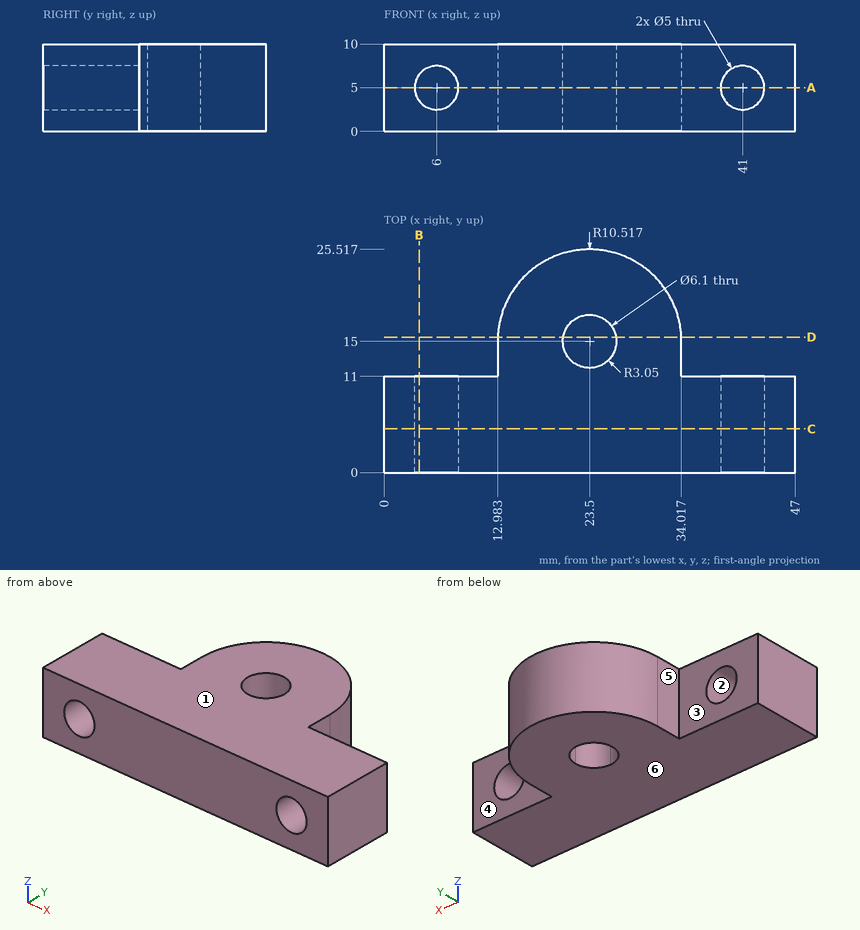
Geometry check sheet. Reference: drawing and pictorial views, mm from the part's lowest x, y, z. A direction names the side the tool comes from. Give positions to 0.01 mm unless a question says otherwise; leave off trailing zeros. Order: outer loops, then holes, each group sorted by start corner. A loop starts at its lowest first (then second) coordinate and runs counter-clockwise, first axis right, second up. Notation, with made-up numbers: (31.25, 68) -> (61.25, 68) arc R11 ccw to (61.25, 88) -> close; hole circle Ø2 at (12, -14). An arc over 180 degrees is marked (long way). Use CSV: the item, a comma, the result in double quotes. Start each with the question number.
1) Sectioned sample at D-D, the plane y = 15.5. Record the boundary of the cut face in (x, z) (1 decimal), plus the area to 3 significant figures.
2) Material ranges on line 1 (X direction, y = 8, z = 5); line 2 (X direction, y = 15, z = 7.25); line 3 (Y direction, x = 23.5, z = 8.25), recorded low to high. Write a range as from..to.
3) Sectioned sample at A-A, the plane z = 5. Give the number of separate pieces and of enclosed holes in the cut face, plus the area to 3 significant figures.
4) Sectioned sample at C-C, the plane y = 5. Record the boundary of the cut face in (x, z).
5) Mould release check, pull along Z, two halves, no side actions. Record for the marked faces 1, 2 and 3: released by +Z, released by -Z, zero draft, split by the parting line, or undercut.
6) Set-up check for the marked faces 4, 5 and 6: record each of +Z, -Z, +X, -X, +Y, -Y from which the full face is reachable in a straight line by a thin tool's end or side.
7) Go/stop test with flat-tipped pins: P1, Ø1.5, axis at y = 17, z = 4, coming from the -X side; P2, Ø5, axis at x = 43, z = 7.5, coming from the +Y side; P3, Ø2, axis at y = 12.5, z = 5.5, coming from the -X side. Record where each tip stops, or that it passes through.
8) Sectioned sample at B-B, the plane x = 4. Record the boundary of the cut face in (y, z), plus the area to 3 significant figures.
Recorded:
1,outline,"(13, 0) -> (20.5, 0) -> (20.5, 10) -> (13, 10) -> close; (26.5, 0) -> (34, 0) -> (34, 10) -> (26.5, 10) -> close"
1,area,"150 mm2"
2,line 1,"0..3.5, 8.5..38.5, 43.5..47"
2,line 2,"12.98..20.45, 26.55..34.02"
2,line 3,"0..11.95, 18.05..25.52"
3,separate pieces,"3"
3,enclosed holes,"1"
3,area,"636 mm2"
4,outline,"(0, 0) -> (47, 0) -> (47, 10) -> (0, 10) -> close; hole circle Ø5 at (6, 5); hole circle Ø5 at (41, 5)"
5,face 1,"released by +Z"
5,face 2,"undercut"
5,face 3,"zero draft"
6,face 4,"+Z, -Z, +X, +Y"
6,face 5,"+Z, -Z, -X, +Y"
6,face 6,"-Z, +X, -X, +Y, -Y"
7,P1,"x = 13.06"
7,P2,"y = 11"
7,P3,"x = 12.98"
8,outline,"(0, 0) -> (11, 0) -> (11, 3.5) -> (0, 3.5) -> close; (0, 6.5) -> (11, 6.5) -> (11, 10) -> (0, 10) -> close"
8,area,"77.0 mm2"
